```python
from build123d import *

# Parameters (mm, degrees)
ESQUISSE1_R                  = 3.125
BOSS_EXTRU_1_DEPTH           = 10
CONG_1_R                     = 1
ESQUISSE2_R                  = 12.5
BOSS_EXTRU_3_DEPTH           = 10
ENL_V_MAT_EXTRU_1_DEPTH      = 21.310096012
ENL_V_MAT_EXTRU_1_DEPTH_BACK = 21.310096012
ESQUISSE6_R                  = 1.45
BOSS_EXTRU_4_DEPTH           = 2
BOSS_EXTRU_4_DEPTH_BACK      = 1
ESQUISSE7_R                  = 0.5
BOSS_EXTRU_5_DEPTH           = 2
BOSS_EXTRU_5_DEPTH_BACK      = 1
ESQUISSE8_R                  = 0.5
CONG_2_R                     = 0.2


with BuildPart() as part:
    # Esquisse1 → Boss.-Extru.1 (new body)
    with BuildSketch(Plane.XY):
        Circle(ESQUISSE1_R)
    extrude(amount=BOSS_EXTRU_1_DEPTH)

    # Congé1
    cong_1_edges = [part.edges().sort_by_distance(p)[0] for p in [
        (-3.125, 0, 10),
    ]]
    fillet(cong_1_edges, radius=CONG_1_R)

    # Esquisse2 → Boss.-Extru.3 (add)
    with BuildSketch(Plane(origin=(0, 0, 0), x_dir=(-1, 0, 0), z_dir=(0, 0, -1))):
        Circle(ESQUISSE2_R)
    extrude(amount=BOSS_EXTRU_3_DEPTH)

    # Esquisse5 → Enlèvement de matière-Révolution1 (revolve, cut)
    with BuildSketch(Plane(origin=(0, 0, 0), x_dir=(0, 0, -1), z_dir=(1, 0, 0)), mode=Mode.PRIVATE) as enl_vement_de_mati_re_r_volution1_sk:
        Polygon((1, 12.5), (1.5, 9.66435909), (3.5, 9.66435909), (4, 12.5), align=None)
        Polygon((6, 12.5), (9, 12.5), (8.5, 9.66435909), (6.5, 9.66435909), align=None)
    revolve(enl_vement_de_mati_re_r_volution1_sk.sketch.rotate(Axis((0, 0, 0), (0, 0, -1)), 90), axis=Axis((0, 0, 0), (0, 0, -1)), mode=Mode.SUBTRACT)

    # Esquisse6 → Enlèv. mat.-Extru.1 (cut, two sides: drawn at the far end of the back side and taken through both)
    with BuildSketch(Plane(origin=(0, 0, 0), x_dir=(1, 0, 0), z_dir=(0, 1, 0)).offset(-ENL_V_MAT_EXTRU_1_DEPTH_BACK)):
        with Locations(Location((0, -5, 0), (0, 0, 270))):
            Circle(ESQUISSE6_R)
    extrude(amount=ENL_V_MAT_EXTRU_1_DEPTH + ENL_V_MAT_EXTRU_1_DEPTH_BACK, mode=Mode.SUBTRACT)

    # Esquisse7 → Boss.-Extru.4 (add, two sides: drawn at the far end of the back side and taken through both)
    with BuildSketch(Plane(origin=(0, 9.66435909, 0), x_dir=(1, 0, 0), z_dir=(0, 1, 0)).offset(-BOSS_EXTRU_4_DEPTH_BACK)):
        with Locations(Location((0, 7.5, 0), (0, 0, 270))):
            Circle(ESQUISSE7_R)
    extrude(amount=BOSS_EXTRU_4_DEPTH + BOSS_EXTRU_4_DEPTH_BACK)

    # Esquisse8 → Boss.-Extru.5 (add, two sides: drawn at the far end of the back side and taken through both)
    with BuildSketch(Plane(origin=(0, -9.66435909, 0), x_dir=(-1, 0, 0), z_dir=(0, -1, 0)).offset(-BOSS_EXTRU_5_DEPTH_BACK)):
        with Locations(Location((0, 2.5, 0), (0, 0, 90))):
            Circle(ESQUISSE8_R)
    extrude(amount=BOSS_EXTRU_5_DEPTH + BOSS_EXTRU_5_DEPTH_BACK)

    # Congé2
    cong_2_edges = [part.edges().sort_by_distance(p)[0] for p in [
        (0, 11.66435909, -8),
        (0, -11.66435909, -2),
    ]]
    fillet(cong_2_edges, radius=CONG_2_R)


solid = part.part
```
Can you work these out from the model? Positions are in its coordinate system, mm. A direction names the side the tool comes from. Give positions to 0.01 mm unless a question says otherwise; leave off trailing zeros. Order: outer loops, then holes, each group sorted by start corner. A loop starts at its lowest first (then second) coordinate and runs counter-clockwise, first axis right, second up. Notation, with made-up numbers: (15, 34) - (32, 34) arc R17 cw to (32, 57) - close; hole circle Ø5 at (68.25, 24.25). An arc over 180 degrees is marked (long way). Use a Markdown table: item, result. Add a question column.
Q1. On a 3-axis mill with a long thin cutter (end or side, diameter ignored), from which of +Z, -Z, +X, -X, +Y, -Y can I reach the whole of each face in a straight line? I mean faces 4 (the cylindrical face through (0, 11, -7)), 5 (the conical face through (-2.13, 9.61, -3.53)), 6 (the cylindrical face through (2.98, 0.94, 4.44)), 7 (the cylindrical face through (0, -11, -2)). Say none if no direction works.
Q2. If we section it at B-B on z = 2.75: Write out the boundary of the cut face in (x, y) (3 decimals), plus the area to 3 significant figures.
Q3. If we section it at C-C on x = 11: Count the separate pieces of the cut face and the enclosed holes in it, plus the area to 3 significant figures.
Q4. I'm going to push flat-ended pins straight in: pin 1 (2 mm diameter, centred on x = 4, z = -4, fed in from +Y); pin 2 (1 mm diameter, centred on x = 8.5, y = -1, fed in from +Z); pin 3 (8 mm diameter, centred on x = 9.5, z = 1.5, fed in from +Y). Where does each tip first touch, or does it pass through?
Q5. If we mould it in two halves opening along X, with no side actions, what happens to faces 1 (the cylindrical face through (-0.555, -0.044, 6.339)), 2 (the cylindrical face through (-11.923, 3.755, -9.493)), 3 (the flat face through (-3, -3, 0))? For each: released by +X, released by -X, zero draft, split by the parting line, or undercut.
Q6. If we section it at A-A on y = 0: Write out the boundary of the cut face in (x, z) (3 decimals), plus the area to 3 significant figures.
Q7. If we section it at D-D on z = 5: Write out the boundary of the cut face in (x, y) (3 decimals), plus the area to 3 significant figures.
Q8. Please list where these lines run through material, in increasing order: line 1 along Z through (x, y) = (0, 1.25); line 2 along Z through (x, y) = (-9.5, -4.25); line 3 along Z through (x, y) = (11.25, 3.75).
Answers follow:
| question | item | result |
|---|---|---|
| 1 | face 4 | +Y |
| 1 | face 5 | none |
| 1 | face 6 | +Z |
| 1 | face 7 | -Y |
| 2 | outline | circle Ø6.25 at (0, 0) |
| 2 | area | 30.7 mm^2 |
| 3 | separate pieces | 3 |
| 3 | enclosed holes | 0 |
| 3 | area | 55.8 mm^2 |
| 4 | pin 1 | stops at y = 12.13 |
| 4 | pin 2 | stops at z = 0 |
| 4 | pin 3 | stops at y = 11.08 |
| 5 | face 1 | undercut |
| 5 | face 2 | split by the parting line |
| 5 | face 3 | zero draft |
| 6 | outline | (-12.5, -10) - (12.5, -10) - (12.5, -9) - (9.664, -8.5) - (9.664, -6.5) - (12.5, -6) - (12.5, -4) - (9.664, -3.5) - (9.664, -1.5) - (12.5, -1) - (12.5, 0) - (3.125, 0) - (3.125, 9) arc R1 ccw to (2.125, 10) - (-2.125, 10) arc R1 ccw to (-3.125, 9) - (-3.125, 0) - (-12.5, 0) - (-12.5, -1) - (-9.664, -1.5) - (-9.664, -3.5) - (-12.5, -4) - (-12.5, -6) - (-9.664, -6.5) - (-9.664, -8.5) - (-12.5, -9) - close; hole circle Ø2.9 at (0, 5) |
| 6 | area | 277 mm^2 |
| 7 | outline | (-1.45, -2.768) - (-1.45, 2.768) arc R3.125 ccw to start; (1.45, -2.768) arc R3.125 ccw to (1.45, 2.768) - close |
| 7 | area | 13.2 mm^2 |
| 8 | line 1 | z = -10 to 3.55, 6.45 to 10 |
| 8 | line 2 | z = -10 to -8.63, -6.37 to -3.63, -1.37 to 0 |
| 8 | line 3 | z = -10 to -8.89, -6.11 to -3.89, -1.11 to 0 |
